from build123d import *

# Parameters (mm, degrees)
F0_W     = 78
F0_H     = 43
F0_W_2   = 66
F0_H_2   = 37
F1_DEPTH = 19
F2_R     = 1.5
F3_DEPTH = 78
F5_DEPTH = 3
F7_DEPTH = 3


with BuildPart() as f1:
    # F0 (on Front) → F1 (new body)
    with BuildSketch(Plane.XZ):
        with Locations((12.482391, -0.926793)):
            Rectangle(F0_W, F0_H)
        with Locations((12.482391, -0.926793)):
            Rectangle(F0_W_2, F0_H_2, mode=Mode.SUBTRACT)
    extrude(amount=F1_DEPTH)

    # F2 (on face) → F3 (cut)
    with BuildSketch(Plane.YZ.offset(51.482391)):
        with Locations((-9.5, 8.573207)):
            Circle(F2_R)
        with Locations((-9.5, -10.426793)):
            Circle(F2_R)
    extrude(amount=-F3_DEPTH, mode=Mode.SUBTRACT)

    # F4 (on face) → F5 (cut)
    with BuildSketch(Plane.YZ.offset(-20.517609)):
        Polygon((-6.646372, 9.966096), (-9.279464, 11.740966), (-12.133092, 10.348076), (-12.353628, 7.180317), (-9.720536, 5.405448), (-6.866908, 6.798337), align=None)
        Polygon((-7.610832, -7.874466), (-10.765796, -7.514562), (-12.654965, -10.066889), (-11.389168, -12.979121), (-8.234204, -13.339025), (-6.345035, -10.786698), align=None)
    extrude(amount=-F5_DEPTH, mode=Mode.SUBTRACT)

    # F6 (on face) → F7 (cut)
    with BuildSketch(Plane(origin=(45.482391, 0, 0), x_dir=(0, -1, 0), z_dir=(-1, 0, 0))):
        Polygon((9.609124, 5.399656), (12.302937, 7.080935), (12.193814, 10.254486), (9.390876, 11.746758), (6.697063, 10.065478), (6.806186, 6.891927), align=None)
        Polygon((9.398182, -13.600587), (12.197677, -12.101867), (12.299495, -8.928073), (9.601818, -7.253), (6.802323, -8.75172), (6.700505, -11.925514), align=None)
    extrude(amount=-F7_DEPTH, mode=Mode.SUBTRACT)


solid = f1.part
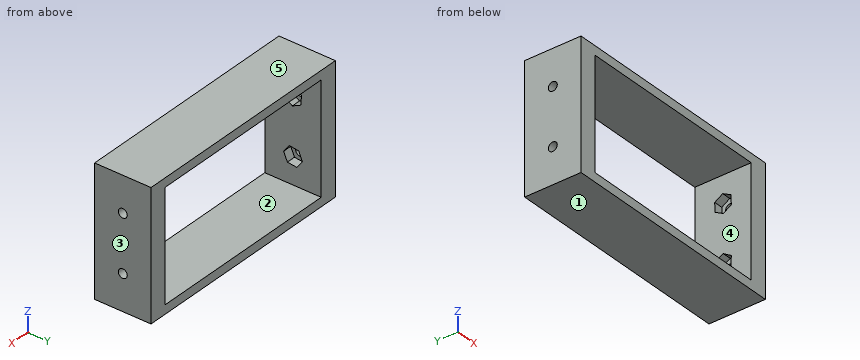
Check sheet for the modelled part. Datum: model origin and axes. Units: mm. Face numbers are marked on the shaded views. A direction names the side the tool comes from. Round coordinates to 2 decimals unless told otherwise and drop trailing zeros. Order: outer loops, then holes, each group sorted by start corner. A loop starts at its lowest first (then second) coordinate and runs counter-clockwise, first axis right, second up.
Q1. Draft check along X on the marked faces 1, 2 and 3. Enter one of: pulls with the +X half, pulls with the -X half, needs draft (parallel to the pull), parting line crosses it, or undercut.
Filled sheet:
face 1: needs draft
face 2: undercut
face 3: pulls with the +X half
Q2. Cross-section at C-C, the plane y = -4.75. Enter the section's corners in (x, z), plus the area to 3 significant figures.
Filled sheet:
outline: (-26.52, -22.43) - (51.48, -22.43) - (51.48, 20.57) - (-26.52, 20.57) - close; hole (-20.52, -19.43) - (45.48, -19.43) - (45.48, 17.57) - (-20.52, 17.57) - close
area: 912 mm2
Q3. Cross-section at A-A, the plane z = 12.5. Enter the section's corners in (x, y).
Filled sheet:
outline: (-26.52, -19) - (-20.52, -19) - (-20.52, 0) - (-26.52, 0) - close; (45.48, -19) - (51.48, -19) - (51.48, 0) - (45.48, 0) - close
Q4. Scan lines: L1, parallel to Z at x = -24.8, y = -9.5; L2, parallel to Z at x = -7, y = -5.5; L3, parallel to X at y = -16.5, z = 16. Record each from-to range of solid material in increasing order.
Filled sheet:
L1: z = -22.43 to -11.93, -8.93 to 7.07, 10.07 to 20.57
L2: z = -22.43 to -19.43, 17.57 to 20.57
L3: x = -26.52 to -20.52, 45.48 to 51.48
Q5. Set-up check for the marked faces 4 and 5: record each of +Z, -Z, +X, -X, +Y, -Y from which the full face is reachable in a straight line by a thin tool's end or side.
Filled sheet:
face 4: +Y, -Y
face 5: +Z, +X, -X, +Y, -Y
Q6. Cross-section at B-B, the plane x = 25.5. Enter the section's corners in (y, z), plus the area to 3 significant figures.
Filled sheet:
outline: (-19, -22.43) - (0, -22.43) - (0, -19.43) - (-19, -19.43) - close; (-19, 17.57) - (0, 17.57) - (0, 20.57) - (-19, 20.57) - close
area: 114 mm2
